from build123d import *

# Parameters (mm, degrees)
F0_R     = 6.25
F0_R_2   = 11
F1_DEPTH = 7
F2_R     = 2


with BuildPart() as f1:
    # F0 (on Front) → F1 (new body)
    with BuildSketch(Plane.XZ):
        with BuildLine():
            ThreePointArc((-9.448443, -32.250276), (7.583595, -15.214765), (31.439673, -11.870146))
            ThreePointArc((31.439673, -11.870146), (43.248737, -2.65025), (32.65378, 7.942547))
            ThreePointArc((32.65378, 7.942547), (9.384576, 14.174969), (-5.439988, 33.162628))
            ThreePointArc((-5.439988, 33.162628), (-19.329184, 38.77963), (-23.205337, 24.307729))
            ThreePointArc((-23.205337, 24.307729), (-16.968171, 1.039797), (-25.999684, -21.292482))
            ThreePointArc((-25.999684, -21.292482), (-23.919553, -36.12938), (-9.448443, -32.250276))
        make_face()
        with Locations((-18.399214, -27.791163)):
            Circle(F0_R, mode=Mode.SUBTRACT)
        Circle(F0_R_2, mode=Mode.SUBTRACT)
        with Locations((33.26746, -2.038605)):
            Circle(F0_R, mode=Mode.SUBTRACT)
        with Locations((-14.868246, 29.829768)):
            Circle(F0_R, mode=Mode.SUBTRACT)
    extrude(amount=F1_DEPTH)

    # F2
    f2_edges = [f1.edges().sort_by_distance(p)[0] for p in [
        (-16.968171, -7, 1.039797),
        (7.583595, 0, -15.214765),
    ]]
    fillet(f2_edges, radius=F2_R)


solid = f1.part
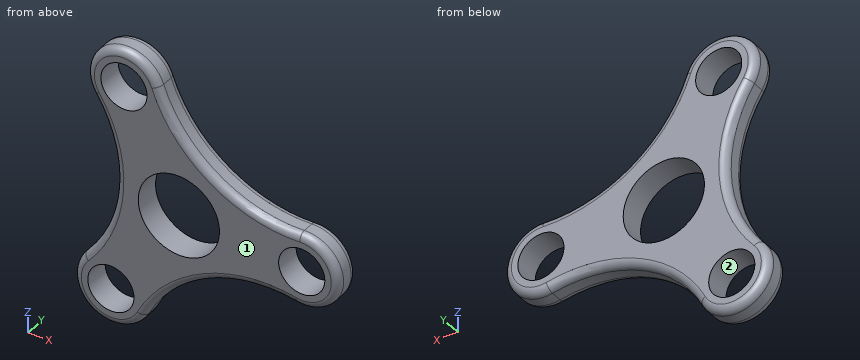
Verification items for the finished model (mm, model axes). Face numbers are marked on the shaded views. Round coordinates to 2 decimals unless told otherwise and drop trailing zeros. Loops run counter-clockwise (first coordinate to the right, second up) from the corner with the lowest first, then second, coordinate; pieces in that order, holes last. Notation, with made-up numbers: (81.25, 36) - (117.25, 36) arc R33 cw to (117.25, 65) - close; hole circle Ø1 at (25.25, 57.5). An arc over 180 degrees is marked (long way). Write item = value, one per line.
Q1. Depth check by flat-ended pin: pin 1 (1.5 mm diameter, centred on y = -1, z = 4.5, fed in from +X); pin 2 (1.5 mm diameter, centred on x = 35.5, y = -6, fed in from +Z); pin 3 (4 mm diameter, centred on y = -2, z = 13.5, fed in from -X); pin 4 (1 mm diameter, centred on y = -4.5, z = -27.5, fed in from -X). Enter the tip coordinate at first touch or a pass-through.
Here are the results:
pin_1 = 41.23
pin_2 = 7.76
pin_3 = -18.89
pin_4 = -28.4
Q2. Sectioned sample at B-B on z = 0. State how many separate pieces and enclosed holes the cut face has, plus the area to 3 significant figures.
Here are the results:
separate_pieces = 3
enclosed_holes = 0
area = 181 mm^2
Q3. Material ranges on L1, parallel to Z at x = -23, y = -3; L2, parallel to X at y = -6.25, z = -4; L3, parallel to X at y = -3, z = -6, recorded low to high.
Here are the results:
L1 = -36.67 to -32.02, -23.56 to -17.27, 23.99 to 35.65
L2 = -17.17 to -10.25, 10.25 to 27.33, 39.2 to 42.63
L3 = -18.07 to -9.22, 9.22 to 28.43, 38.1 to 42.45
Q4. Sectioned sample at A-A on y = -3. Record the boundary of the cut face in (x, z), plus the area to 3 significant figures.
Here are the results:
outline = (-26, -21.29) arc R10 ccw (long way) to (-9.45, -32.25) arc R37.93 cw to (31.44, -11.87) arc R10 ccw (long way) to (32.65, 7.94) arc R37.93 cw to (-5.44, 33.16) arc R10 ccw (long way) to (-23.21, 24.31) arc R37.93 cw to start; hole circle Ø12.5 at (-18.4, -27.79); hole circle Ø12.5 at (-14.87, 29.83); hole circle Ø22 at (0, 0); hole circle Ø12.5 at (33.27, -2.04)
area = 1,730 mm^2
Q5. Mould release check, pull along Z, two halves, no side actions. Record for the marked faces 1 and 2: +Z half, -Z half, draft (parallel to the pull), parting line (faces both ways), or undercut.
Here are the results:
face_1 = draft
face_2 = undercut
